```python
from build123d import *

# Parameters (mm, degrees)
F1_DEPTH     = 6
F2_T1_DEPTH  = 157.6354832979
F3_T1_DEPTH  = 180.911939444
F3_T3_DEPTH  = 11.1833176621
F3_T8_DEPTH  = 154.2537676368
F3_T13_DEPTH = 154.2537676368
F4_T1_DEPTH  = 108.3530023153


# Not quite as in the source:
# - a fillet or chamfer that OpenCascade refuses, or shapes differently, is made with other operations: its cross-section is extruded or revolved along the edge and cut away or added


with BuildPart() as f1:
    # F0 (on Top) → F1 (new body)
    with BuildSketch(Plane.XY):
        Polygon((38.1666665349, 7), (-81.8333334651, 7), (-81.8333334651, 0), (38.5162681341, 0), align=None)
        with BuildLine():
            Line((39.3004275709, 10), (38.1666665349, 7))
            Line((38.1666665349, 7), (38.5162681341, 0))
            Line((38.5162681341, 0), (46.4909672737, 0))
            Line((46.4909672737, 0), (77.9909640551, 0))
            Line((77.9909640551, 0), (77.5119066238, 1.5898427228))
            add(Edge.make_bspline(
                [(46.4909672737, 10), (49.5646846807, 9.1582136368), (54.0969093449, 5.5068681922), (67.4802237728, 4.9316783562), (74.0574866156, 2.5085939236), (77.5119066238, 1.5898427228)],
                knots=[0, 0, 0, 0, 0.3024831153, 0.6658844955, 1, 1, 1, 1], degree=3))
            Line((46.4909672737, 10), (39.3004275709, 10))
        make_face()
        Polygon((-81.8333334651, 0), (-81.8333334651, 7), (-108.5871011019, 7), (-111.7533296347, 0), align=None)
    extrude(amount=F1_DEPTH)

    # F2: chamfer of 30 x 2.8 on 2 edges, made by hand

    # F2_s2 → F2_t1 (cut)
    with BuildSketch(Plane(origin=(28.992055027, -96.2156198783, 0), x_dir=(0, 0, 1), z_dir=(-0.2885105142, 0.9574767272, 0))):
        Polygon((3.2, 74.6745330178), (6, 44.6745330178), (6, 74.6745330178), align=None)
        Polygon((2.8, 74.6745330178), (0, 44.6745330178), (0, 74.6745330178), align=None)
    extrude(amount=F2_T1_DEPTH, mode=Mode.SUBTRACT)

    # F3: fillet of radius 1.5 on 5 edges, made by hand

    # F3_s2 → F3_t1 (cut)
    with BuildSketch(Plane.YZ.offset(-115.5033296347)):
        with BuildLine():
            ThreePointArc((1.5, 6), (0.4393398282, 5.5606601718), (0, 4.5))
            Line((0, 4.5), (0, 6))
            Line((0, 6), (1.5, 6))
        make_face()
        with BuildLine():
            ThreePointArc((1.5, 0), (0.4393398282, 0.4393398282), (0, 1.5))
            Line((0, 1.5), (0, 0))
            Line((0, 0), (1.5, 0))
        make_face()
    extrude(amount=F3_T1_DEPTH, mode=Mode.SUBTRACT)

    # F3_s4 → F3_t3 (cut)
    with BuildSketch(Plane.XY.offset(-2.591658831)):
        with BuildLine():
            ThreePointArc((38.9339491071, 9.0302759078), (39.4842763115, 9.7339801177), (40.3370911034, 10))
            Line((40.3370911034, 10), (39.3004275709, 10))
            Line((39.3004275709, 10), (38.9339491071, 9.0302759078))
        make_face()
    extrude(amount=F3_T3_DEPTH, mode=Mode.SUBTRACT)


with BuildPart() as f3_tool6:
    # F3_s7 → F3_t8 (new body)
    with BuildSketch(Plane.YZ.offset(41.9166665349)):
        with BuildLine():
            ThreePointArc((7, 4.5), (6.5606601718, 5.5606601718), (5.5, 6))
            Line((5.5, 6), (7, 6))
            Line((7, 6), (7, 4.5))
        make_face()
    extrude(amount=-F3_T8_DEPTH)

    split(bisect_by=Plane(origin=(31.0819782613, -11.7465119587, 0), x_dir=(0, 0, 1), z_dir=(-0.9354279975, 0.3535172719, 0)), keep=Keep.TOP)


with BuildPart() as f1_1:
    add(f1.part)

    # F3_t5: cut F3_tool6
    add(f3_tool6.part, mode=Mode.SUBTRACT)


with BuildPart() as f3_tool11:
    # F3_s12 → F3_t13 (new body)
    with BuildSketch(Plane.YZ.offset(41.9166665349)):
        with BuildLine():
            ThreePointArc((7, 1.5), (6.5606601718, 0.4393398282), (5.5, 0))
            Line((5.5, 0), (7, 0))
            Line((7, 0), (7, 1.5))
        make_face()
    extrude(amount=-F3_T13_DEPTH)

    split(bisect_by=Plane(origin=(31.0819782613, -11.7465119587, 0), x_dir=(0, 0, 1), z_dir=(-0.9354279975, 0.3535172719, 0)), keep=Keep.TOP)


with BuildPart() as f1_2:
    add(f1_1.part)

    # F3_t10: cut F3_tool11
    add(f3_tool11.part, mode=Mode.SUBTRACT)

    # F4: chamfer of 20 x 2.8 on 2 edges, made by hand

    # F4_s2 → F4_t1 (cut)
    with BuildSketch(Plane(origin=(4.9298048814, 10.8989713826, 0), x_dir=(0, 0, 1), z_dir=(-0.4121205293, -0.9111293373, 0))):
        Polygon((6, 81.8217371748), (3.2, 101.8217371748), (6, 101.8217371748), align=None)
        Polygon((0, 81.8217371748), (2.8, 101.8217371748), (0, 101.8217371748), align=None)
    extrude(amount=F4_T1_DEPTH, mode=Mode.SUBTRACT)


solid = f1_2.part
```
CAD build for the part. Positions are in the model's coordinates, mm. A direction names the side the tool comes from. Round coordinates to 2 decimals unless told otherwise and drop trailing zeros. Loops run counter-clockwise (first coordinate to the right, second up) from the corner with the lowest first, then second, coordinate; pieces in that order, holes last. Notation, with made-up numbers: M 63,-28 L 67,-28 A32 cw 67,11 Z; hole C -36,52 d9. An arc over 180 degrees is marked long. Use a Markdown table: item, result. Add a question column.
(1) Cut at A-A (x = 29.5). Give the cut face in (y, z), and give its area (3 significant figures).
(2) Drill centre lines: line 1 (Y direction, x = -83, z = 2.25); line 2 (Z direction, x = 7, y = 5.75); line 3 (Z direction, x = 4, y = 6.75). Where is each one in solid material? Low to high.
(3) Flat gauge pin, fed straight in: pin 1 (2.5 mm diameter, centred on x = -59, z = 2.5, fed in from +Y). Where does the tip first touch, or does it go through?
(4) Which spindle directions (+Z, -Z, +X, -X, +Y, -Y) get a long thin tool onto all of the face, cutting with end or side? Do faces 1 (the face through (-22, 4, 0)), 2 (the face through (-34, 7, 3)). Say none if no direction does.
Geometry says:
| question | item | result |
|---|---|---|
| 1 | outline | M 0,1.5 A1.5 ccw 1.5,0 L 5.5,0 A1.5 ccw 7,1.5 L 7,4.5 A1.5 ccw 5.5,6 L 1.5,6 A1.5 ccw 0,4.5 Z |
| 1 | area | 40.1 mm² |
| 2 | line 1 | y = 0 to 7 |
| 2 | line 2 | z = 0.02 to 5.98 |
| 2 | line 3 | z = 0.67 to 5.33 |
| 3 | pin 1 | stops at y = 7 |
| 4 | face 1 | -Z, +X, -X, +Y, -Y |
| 4 | face 2 | +Z, -Z, -X, +Y |
